Autodesk Inventor part; units mm, degrees
ref_plane "YZ Plane" through (0, 0, 0) normal (1, 0, 0) x (0, 1, 0)
ref_plane "XZ Plane" through (0, 0, 0) normal (0, 1, 0) x (-1, 0, 0)
ref_plane "XY Plane" through (0, 0, 0) normal (0, 0, 1) x (1, 0, 0)
sketch "草圖1" plane through (0, 0, 0) normal (0, 0, 1) x (1, 0, 0)
  circle A0 centre (0, 0) radius 80
  circle A1 centre (0, 0) radius 70
  circle A2 centre (0, 0) radius 55
  dimension "d0" = 160
  dimension "d1" = 140
  dimension "d2" = 110
extrude "擠出1" add sketch "草圖1" against normal blind 30
sketch "草圖2" plane through (0, 0, -30) normal (0, 0, -1) x (-1, 0, 0)
  circle A0 centre (0, 0) radius 80
extrude "擠出2" add sketch "草圖2" along normal blind 10
sketch "草圖3" plane through (0, 0, -40) normal (0, 0, -1) x (-1, 0, 0)
  circle A0 centre (0, 0) radius 25
  dimension "d7" = 50
extrude "擠出3" add sketch "草圖3" along normal blind 5
properties part number "螺旋鉤子底座"
Design review of the part built by this model. Coordinates are the model's own, in mm. A direction names the side the tool comes from. Round coordinates to 2 decimals unless told otherwise and drop trailing zeros. Write each loop counter-clockwise with the first axis right and the second up, starting at its lowest first coordinate (ties: lowest second). Pieces come first, ordered by that corner, then holes. Notation, with made-up numbers: M -8.75,36.25 L 39.25,36.25 A20 cw 39.25,46.25 Z; hole C 81,31 d11. An arc over 180 degrees is marked long. One line per item, written item: value. Start each with the question number.
1. Take a section at A-A on y = 0. State the section outline as (x, z) points, then the cut area to 3 significant figures.
2. Take a section at C-C on z = -16. State the section outline as (x, y) points, then the cut area to 3 significant figures.
3. Clearance check with flat-ended pins moving along their axes: P1, Ø6, axis at x = -26, y = -11, coming from the -Z side; P2, Ø5, axis at y = -9, z = -33, coming from the -X side; P3, Ø12, axis at y = -60.5, z = -12.5, coming from the +X side. State where each tip first meets the part, or that it passes through.
4. Take a section at D-D on z = -36. State the section outline as (x, y) points.
5. For faces 1 (the face through (-55.55, -42.594, -14.79)), 2 (the face through (0, -71, 0)), 3 (the face through (-17, 19, -40)), list the 3-axis set-ups (+Z, -Z, +X, -X, +Y, -Y) from which the entire face can be reached by the end or side of a thin tool; tool diameter is ignored.
6. Draft analysis for pull direction X (two halves, no side actions). For faces 4 (the face through (42, -36, -30)), 5 (the face through (-1, 1, 0)), 6 (the face through (-23.846, -7.509, -42.465)), 7 (the face through (-11.923, -53.692, -14.79)), state which applies: pulls with the +X half, pulls with the -X half, needs draft (parallel to the pull), parting line crosses it, or undercut.
7. To check wall thickness, follow probe 1 along Y at (x, z) = (0, -9.25); probe 2 along X at (y, z) = (-44.5, -9); probe 3 along X at (y, z) = (-30, -21). State the ranges of each line that lie inside material, in increasing order. Write a range as from..to.
Computed:
1. outline: M -80,-40 L -25,-40 L -25,-45 L 25,-45 L 25,-40 L 80,-40 L 80,0 L 70,0 L 70,-30 L 55,-30 L 55,0 L -55,0 L -55,-30 L -70,-30 L -70,0 L -80,0 Z
1. area: 5,750 mm²
2. outline: C 0,0 d160; C 0,0 d110; hole C 0,0 d140
2. area: 14,200 mm²
3. P1: stops at z = -40
3. P2: stops at x = -79.74
3. P3: stops at x = 58.56
4. outline: C 0,0 d160
5. face 1: +Z
5. face 2: +Z, +X, -X, +Y, -Y
5. face 3: -Z
6. face 4: undercut
6. face 5: needs draft
6. face 6: parting line crosses it
6. face 7: undercut
7. probe 1: y = -80..-70, -55..55, 70..80
7. probe 2: x = -66.48..-54.03, -32.32..32.32, 54.03..66.48
7. probe 3: x = -74.16..-63.25, -46.1..46.1, 63.25..74.16
